from build123d import *

# Parameters (mm, degrees)
SKETCH_2_W          = 80
SKETCH_2_H          = 40
EXTRUDE_1_DEPTH     = 10
FILLET_3_R          = 20
CUT_EXTRUDE_6_REACH = 50.99
SKETCH_8_R          = 10
SKETCH_9_R          = 8
EXTRUDE_2_DEPTH     = 6


with BuildPart() as part:
    # 草图2 → 凸台-拉伸1 (new, symmetric)
    with BuildSketch(Plane.XY):
        Rectangle(SKETCH_2_W, SKETCH_2_H)
    extrude(amount=EXTRUDE_1_DEPTH, both=True)

    # 圆角3
    fillet_3_edges = [part.edges().sort_by_distance(p)[0] for p in [
        (40, -20, 0),
        (40, 20, 0),
    ]]
    fillet(fillet_3_edges, radius=FILLET_3_R - 0.0001)  # a hair under: the kernel refuses the full size

    # 草图8 → 切除-拉伸6 (cut, up to next)
    with BuildSketch(Plane(origin=(0, 0, -10), x_dir=(-1, 0, 0), z_dir=(0, 0, -1)), mode=Mode.PRIVATE) as cut_extrude_6_sk1:
        with Locations((-20, 0)):
            Circle(SKETCH_8_R)
    cut_extrude_6_tool1 = extrude(cut_extrude_6_sk1.sketch, amount=-CUT_EXTRUDE_6_REACH, mode=Mode.PRIVATE) & part.part
    add(cut_extrude_6_tool1.solids().sort_by_distance((20, 0, -10))[0], mode=Mode.SUBTRACT)

    # 草图9 → 凸台-拉伸2 (add)
    with BuildSketch(Plane.ZY.offset(40)):
        Circle(SKETCH_9_R)
    extrude(amount=EXTRUDE_2_DEPTH)


solid = part.part
Verification items for the finished model (mm, model axes). A direction names the side the tool comes from. Coordinates: 2 decimals unless noted, no trailing zeros. Write each loop counter-clockwise with the first axis right and the second up, starting at its lowest first coordinate (ties: lowest second). Pieces come first, ordered by that corner, then holes. Notation, with made-up numbers: M 32.25,12 L 50.25,12 A20 ccw 50.25,44 Z; hole C 46.5,26 d11. An arc over 180 degrees is marked long. One line per question, with ' | ' between items.
1) Sectioned sample at B-B on x = 23.5. Record the cut outline in (y, z).
Solutions:
outline: M -19.69,-10 L -9.37,-10 L -9.37,10 L -19.69,10 Z; M 9.37,-10 L 19.69,-10 L 19.69,10 L 9.37,10 Z
2) Sectioned sample at D-D on y = 4.5. Record the cut outline in (x, z).
Solutions:
outline: M -46,-6.61 L -40,-6.61 L -40,-10 L 11.07,-10 L 11.07,10 L -40,10 L -40,6.61 L -46,6.61 Z; M 28.93,-10 L 39.49,-10 L 39.49,10 L 28.93,10 Z
3) Material ranges on L1, parallel to Y at x = 20, z = -3.5; L2, parallel to X at y = -0.5, z = -3.5; L3, parallel to X at y = 8, z = 5.5, recorded low to high.
Solutions:
L1: -20 to -10, 10 to 20 | L2: -46 to 10.01, 29.99 to 39.99 | L3: -40 to 14, 26 to 38.33
4) Sectioned sample at C-C on y = -4. Record the cut outline in (x, z).
Solutions:
outline: M -46,-6.93 L -40,-6.93 L -40,-10 L 10.83,-10 L 10.83,10 L -40,10 L -40,6.93 L -46,6.93 Z; M 29.17,-10 L 39.6,-10 L 39.6,10 L 29.17,10 Z
5) Depth check by flat-ended pin: pin 1 Ø4 at (y, z) = (15.5, -0.5) entering from -X. Enter the tip coordinate at first touch or a pass-through.
Solutions:
pin 1: x = -40
6) Access from +Z, -Z, +X, -X, +Y, -Y to the whole of each face (thin tool, end or side, straight path). Record for faces 5 (the face through (-10, 20, 0)), 6 (the face through (-42.96, -7.81, -1.73)).
Solutions:
face 5: +Z, -Z, +X, -X, +Y | face 6: -X
7) Release check for a two-part mould opening along Y. For faces 1 (the face through (34.297, 13.986, -0.14)), 2 (the face through (34.297, -13.986, 0.14)), 3 (the face through (-1, 0, -10)), 4 (the face through (10.46, 3, -0.14)) record: +Y half, -Y half, draft (parallel to the pull), parting line (faces both ways), or undercut.
Solutions:
face 1: +Y half | face 2: -Y half | face 3: draft | face 4: undercut
